Build history of the part. All positions in model axes, mm. Face numbers are marked on the shaded views. Give positions to 0.01 mm unless a question says otherwise; leave off trailing zeros. Loops run counter-clockwise (first coordinate to the right, second up) from the corner with the lowest first, then second, coordinate; pieces in that order, holes last. Notation, with made-up numbers: (-36, -33) - (-4, -33) arc R27 cw to (-4, -6) - close; hole circle Ø7 at (4.25, 25). An arc over 180 degrees is marked (long way). Return JSON: item names as keys, results as strings. Group by question number.
1) Drill centre lines: probe 1 along Y at (x, z) = (-10, 44.5) (1 decimal); probe 2 along Z at (x, y) = (0, 4); probe 3 along Z at (x, y) = (0, 16.75). Where is each one in solid material? Low to high. Write a range as from..to.
2) Mould opens along X. For the marked faces 1, 2 and 3 say: released by +X, released by -X, zero draft, split by the parting line, or undercut.
3) Slice it at A-A (y = 15.5). List the corners of the cut face in (x, z) (1 decimal), and give its area (3 significant figures).
4) Drop flat-ended pins along their axis: pin 1 (5 mm diameter, centred on x = -17.5, y = 8, fed in from +Z); pin 2 (12 mm diameter, centred on x = 21, y = 32.5, fed in from +Z); pin 3 (2 mm diameter, centred on y = 36, z = 38.5, fed in from +X); pin 4 (3 mm diameter, centred on x = 9, z = -38.5, fed in from -Y). Give the stop position or say it passes through.
5) Slice it at B-B (y = 32). List the corners of the cut face in (x, z).
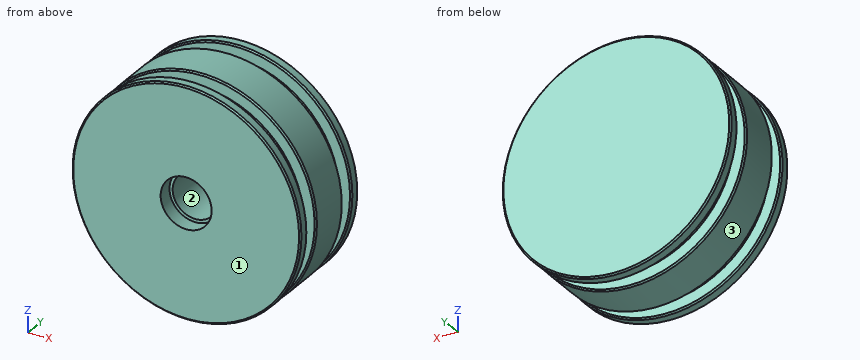
Autodesk Inventor part; units mm, degrees
ref_plane "YZ Plane" through (0, 0, 0) normal (1, 0, 0) x (0, 1, 0)
ref_plane "XZ Plane" through (0, 0, 0) normal (0, 1, 0) x (-1, 0, 0)
ref_plane "XY Plane" through (0, 0, 0) normal (0, 0, 1) x (1, 0, 0)
sketch "Sketch1" plane through (0, 0, 0) normal (0, 0, 1) x (1, 0, 0)
  line L0 (50.8, 0) -> (50.8, 39.0312) construction
  line L1 (0, 0) -> (49.8475, 0)
  line L2 (44.45, 0) -> (44.45, 51.6727)
  line L3 (0, 0) -> (0, 50.5742)
  line L4 (49.8475, 0) -> (49.8475, 45.6895)
  line L5 (49.8475, 4.7625) -> (44.45, 4.7625)
  line L6 (44.45, 11.1125) -> (49.8475, 11.1125)
  line L7 (49.8475, 30.1625) -> (44.45, 30.1625)
  line L8 (44.45, 36.5125) -> (49.8475, 36.5125)
  line L9 (49.8475, 41.275) -> (0, 41.275)
  point P0 (47.1487, 36.5125)
  point P1 (44.45, 30.1625)
  dimension "d1" = 49.8475
  dimension "d2" = 44.45
  dimension "d3" = 6.35
  dimension "d4" = 6.35
  dimension "d5" = 4.7625
  dimension "d6" = 19.05
  dimension "d7" = 4.7625
  dimension "d12" = 41.275
revolve "Revolution1" add sketch "Sketch1" angle 360 about axis through (0, 0, 0) along (0, 1, 0) contours L3 L9 L2 L1 | L2 L5 L4 L1 | L9 L4 L8 L2 | L2 L7 L4 L6
chamfer "Chamfer1" distance 0.635 angle 45 6 edges at (-49.8475, 0, 0) (-49.8475, 4.7625, 0) (-49.8475, 11.1125, 0) (-49.8475, 30.1625, 0) (-49.8475, 36.5125, 0) (-49.8475, 41.275, 0)
sketch "Sketch2" plane through (0, 0, 0) normal (0, -1, 0) x (1, 0, 0)
  circle A0 centre (0, 0) radius 9.7409
  circle A1 centre (0, 0) radius 11.1125
  dimension "d16" = 19.4818
  dimension "d17" = 22.225
extrude "Extrusion1" cut sketch "Sketch2" against normal up to surface (30.1625 mm away) contours A0
extrude "Extrusion2" cut sketch "Sketch2" against normal blind 6.35 contours A0 | A1
properties part number "2 Piston"
Results:
{
 "1": {"probe 1": "0..4.8, 11.1..30.2, 36.5..41.3", "probe 2": "-49.85..-11.11, 11.11..49.85", "probe 3": "-49.85..-9.74, 9.74..49.85"},
 "2": {"face 1": "zero draft", "face 2": "undercut", "face 3": "split by the parting line"},
 "3": {"outline": "circle Ø99.7 at (0, 0); hole circle Ø19.5 at (0, 0)", "area": "7,510 mm2"},
 "4": {"pin 1": "z = 41.84", "pin 2": "z = 47.28", "pin 3": "x = 31.84", "pin 4": "y = 0"},
 "5": {"outline": "circle Ø88.9 at (0, 0)"}
}
